Study the drawing (mm; zero at the part's minimum x, y, z) and answer. A direction names the side the tool comes from. Coordinates: 2 decimals unless noted, no trailing zeros. Write each loop counter-clockwise with the first axis right and the second up, starting at its lowest first coordinate (ties: lowest second). Pieces come first, ordered by that corner, then holes. Notation, with made-up numbers: M 39,-25 L 72,-25 A12 cw 72,-18 Z; hole C -22,66.25 d11. An arc over 180 degrees is marked long. Answer as CSV lines item,"result". Start each with the question number.
(1) Find the intervals of material crossed by L1, parallel to Y at x = 8.5, z = 0.7; L2, parallel to Y at x = 8.5, z = 1.7; L3, parallel to Z at x = 14.75, y = 8.75, in increasing order. Write a range as [from, to].
(2) A cutting plane is placed at A-A on x = 8.5. Give the vertices of the cut face in (y, z).
(3) A cutting plane is placed at B-B on y = 8.5. Give the vertices of the cut face in (x, z), then the cut area to 3 significant figures.
(4) A cutting plane is placed at D-D on y = 6.25. Give the vertices of the cut face in (x, z).
(5) For the marked faces 1 and 2, determine the directions among +Z, -Z, +X, -X, +Y, -Y from which every point of the face is accessible in a straight line to the end or side of a thin tool.
(6) A cutting plane is placed at C-C on z = 3.9. Give the vertices of the cut face in (x, y), then the cut area to 3 significant figures.
(7) Flat-ended cylindrical pins translate along their axes: P1, Ø2.5, axis at x = 8.5, y = 8.5, coming from the -Z side; P2, Ø8, axis at x = 15, y = 12, coming from the +Z side; P3, Ø0.8, axis at x = 8.5, y = 4.94, coming from the -Z side; P4, Ø2, axis at y = 7, z = 1, coming from the +X side (1 decimal). Find the tip coordinate at first contact, or state that the pin passes through.
(8) The mould has two halves that part along Y. Classify the marked faces 3, 4 and 5: released by +Y, released by -Y, zero draft, split by the parting line, or undercut.
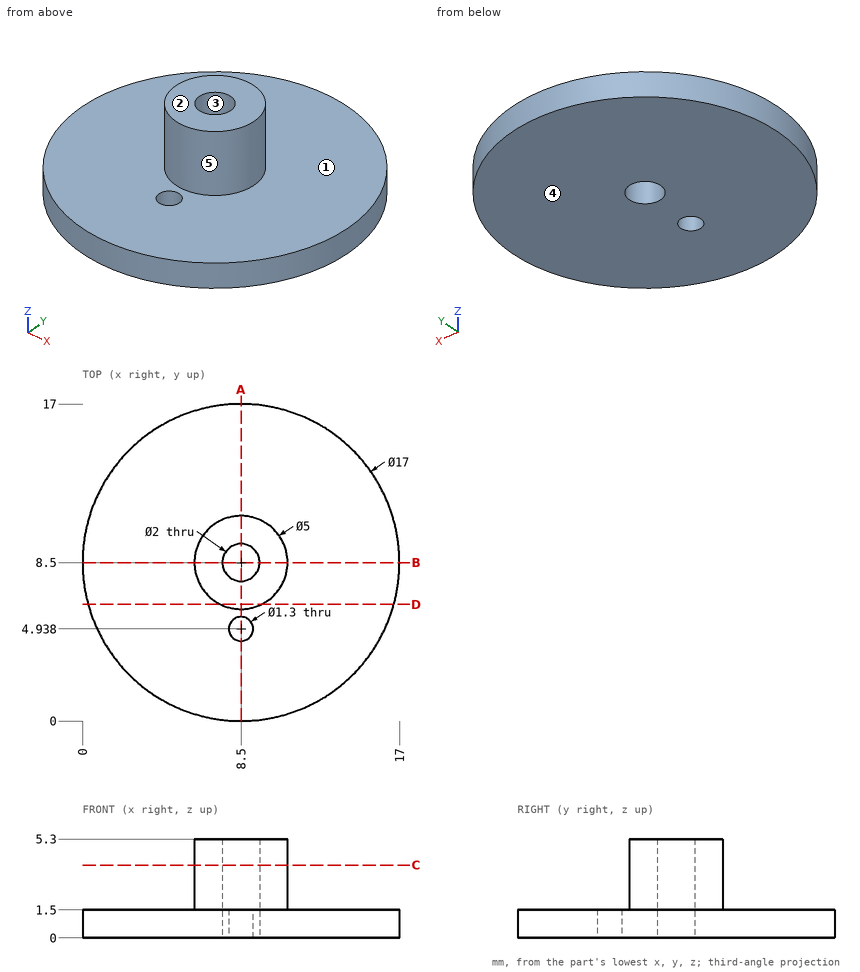
Here are the results:
1,L1,"y = [0, 4.29], [5.59, 7.5], [9.5, 17]"
1,L2,"y = [6, 7.5], [9.5, 11]"
1,L3,"z = [0, 1.5]"
2,outline,"M 0,0 L 4.29,0 L 4.29,1.5 L 0,1.5 Z; M 5.59,0 L 7.5,0 L 7.5,5.3 L 6,5.3 L 6,1.5 L 5.59,1.5 Z; M 9.5,0 L 17,0 L 17,1.5 L 11,1.5 L 11,5.3 L 9.5,5.3 Z"
3,outline,"M 0,0 L 7.5,0 L 7.5,5.3 L 6,5.3 L 6,1.5 L 0,1.5 Z; M 9.5,0 L 17,0 L 17,1.5 L 11,1.5 L 11,5.3 L 9.5,5.3 Z"
3,area,"33.9 mm^2"
4,outline,"M 0.3,0 L 16.7,0 L 16.7,1.5 L 9.59,1.5 L 9.59,5.3 L 7.41,5.3 L 7.41,1.5 L 0.3,1.5 Z"
5,face 1,"+Z"
5,face 2,"+Z, +X, -X, +Y, -Y"
6,outline,"C 8.5,8.5 d5; hole C 8.5,8.5 d2"
6,area,"16.5 mm^2"
7,P1,"stops at z = 0"
7,P2,"stops at z = 1.5"
7,P3,"passes through"
7,P4,"stops at x = 17"
8,face 3,"undercut"
8,face 4,"zero draft"
8,face 5,"split by the parting line"
